Part print with two shaded views. Sizes in mm from the minimum x, y, z corner. A direction names the side the tool comes from. Give positions to 0.01 mm unless a question says otherwise; leave off trailing zeros. Write each loop counter-clockwise with the first axis right and the second up, starting at its lowest first coordinate (ties: lowest second). Pieces come first, ordered by that corner, then holes. Notation, with made-up numbers: (10, -22.75) - (37, -22.75) arc R11 cw to (37, -12.75) - close; hole circle Ø5 at (16.25, -18.5). An arc over 180 degrees is marked (long way). One line per item, written item: value. Start each with the question number.
(1) Cut at C-C, the plane y = 8.25. List the corners of the cut face in (x, z).
(2) Cut at D-D, the plane y = 18.75. List the corners of the cut face in (x, z), and give its area (3 significant figures).
(3) Probe L1, parallel to Z at x = 4, y = 10.25; L2, parallel to Y at x = 4.75, z = 10. List the from-to ranges inside material, lowest first.
(4) 3-axis set-ups, long thin cutter, end or side, ignore diameter. For the marked faces 1 and 2: which of +Z, -Z, +X, -X, +Y, -Y reach the whole face in a straight line?
(5) Drop flat-ended pins along their axis: P1, Ø4, axis at x = 3.5, y = 16.5, coming from the -Z side; P2, Ø4, axis at x = 1.5, y = 13.5, coming from the +Z side; P3, Ø6, axis at x = 6.5, z = 5, coming from the -Y side. Give the stop position or say it passes through.
(6) Cut at B-B, the plane x = 6.75. List the corners of the cut face in (y, z), and give its area (3 significant figures).
(7) Mould opens along Y. For the marked faces 3, 4 and 5 say: pulls with the +Y half, pulls with the -Y half, needs draft (parallel to the pull), parting line crosses it, or undercut.
(8) Cut at A-A, the plane z = 10. List the corners of the cut face in (x, y), and give its area (3 significant figures).
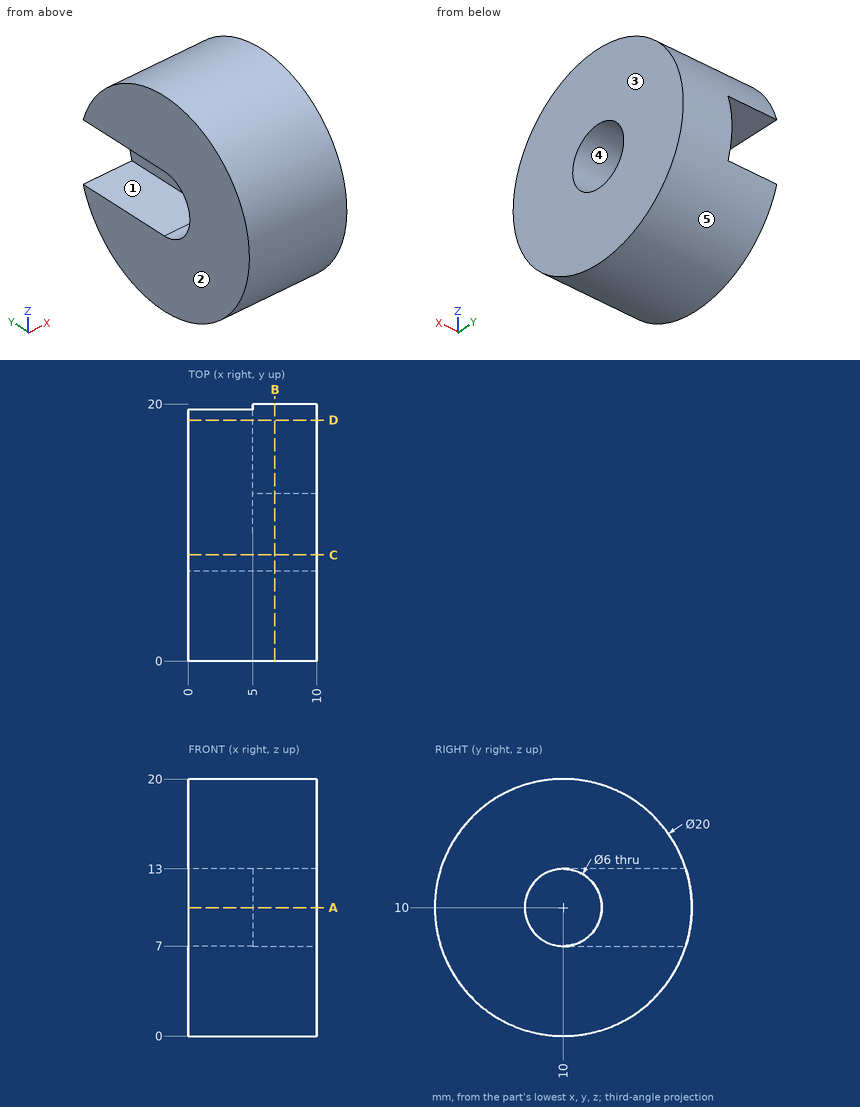
Answers follow:
1. outline: (0, 0.15) - (10, 0.15) - (10, 7.56) - (0, 7.56) - close; (0, 12.44) - (10, 12.44) - (10, 19.85) - (0, 19.85) - close
2. outline: (0, 5.16) - (10, 5.16) - (10, 14.84) - (0, 14.84) - (0, 13) - (5, 13) - (5, 7) - (0, 7) - close
2. area: 66.8 mm²
3. L1: z = 0 to 7, 13 to 20
3. L2: y = 0 to 7
4. face 1: -X, +Y
4. face 2: +Z, -Z, -X, +Y, -Y
5. P1: stops at z = 1.07
5. P2: stops at z = 19.89
5. P3: stops at y = 0.2
6. outline: circle Ø20 at (10, 10); hole circle Ø6 at (10, 10)
6. area: 286 mm²
7. face 3: needs draft
7. face 4: undercut
7. face 5: parting line crosses it
8. outline: (0, 0) - (10, 0) - (10, 7) - (0, 7) - close; (5, 13) - (10, 13) - (10, 20) - (5, 20) - close
8. area: 105 mm²
